Design review of the part shown in the three views and the two pictorial views. Dimensions are in mm from the part's minimum x, y and z. A direction names the side the tool comes from. Give positions to 0.01 mm unless a question says otherwise; leave off trailing zeros. Order: outer loops, then holes, each group sorted by start corner. A loop starts at its lowest first (then second) coordinate and runs counter-clockwise, first axis right, second up. Notation, with made-up numbers: (33.25, -9) - (72.25, -9) arc R11 ccw to (72.25, -2) - close; hole circle Ø3 at (85.25, 61). An arc over 180 degrees is marked (long way). Put each result on its own line as item: value.
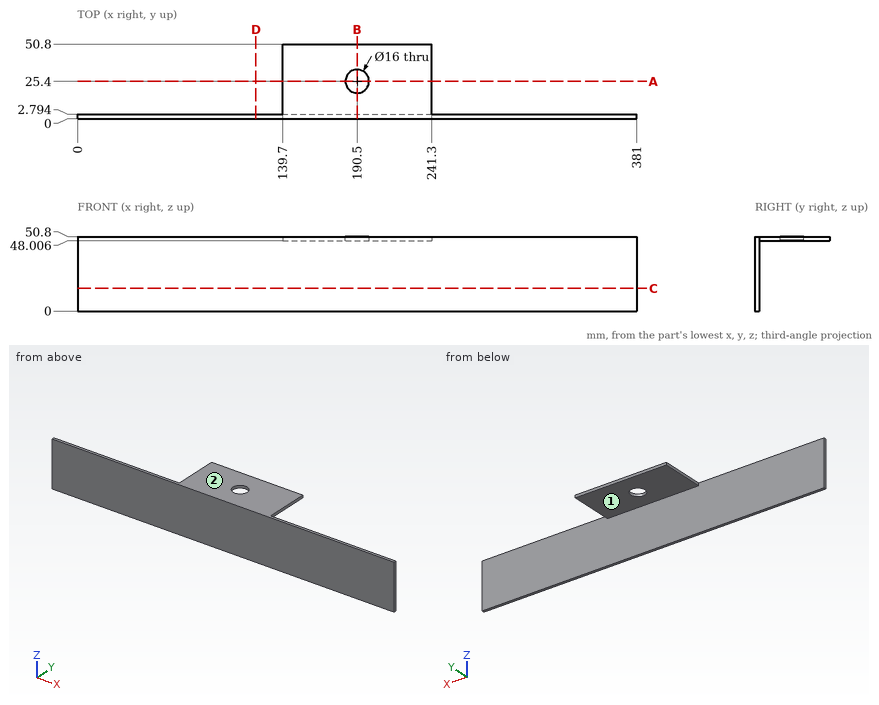
(1) Clearance check with flat-ended pins moving along their axes: pin 1 Ø14.5 at (x, y) = (190.5, 25.4) entering from -Z; pin 2 Ø4 at (x, z) = (326, 21.5) entering from +Y; pin 3 Ø0.8 at (y, z) = (36, 49) entering from +X; pin 4 Ø1.4 at (y, z) = (17.5, 49) entering from -X. State where each tip first meets the part, or that it passes through.
The answers:
pin 1: through
pin 2: y = 2.79
pin 3: x = 241.3
pin 4: x = 139.7
(2) For the marked faces 1 and 2, list the 3-axis set-ups (+Z, -Z, +X, -X, +Y, -Y) from which the entire face can be reached by the end or side of a thin tool; tool diameter is ignored.
The answers:
face 1: -Z, +X, -X, +Y
face 2: +Z, +X, -X, +Y, -Y
(3) Take a section at A-A, the plane y = 25.4. Write out the cut boundary in (x, z), then the cut area to 3 significant figures.
The answers:
outline: (139.7, 48.01) - (182.5, 48.01) - (182.5, 50.8) - (139.7, 50.8) - close; (198.5, 48.01) - (241.3, 48.01) - (241.3, 50.8) - (198.5, 50.8) - close
area: 239 mm^2
(4) Wall thickness on L1, parallel to Y at x = 190, z = 49; L2, parallel to Y at x = 314, z = 12; L3, parallel to Z at x = 219, y = 37: over which ranges is each line inside the solid? List them lowest first.
The answers:
L1: 0 to 17.42, 33.38 to 50.8
L2: 0 to 2.79
L3: 48.01 to 50.8
(5) Take a section at B-B, the plane x = 190.5. Write out the cut boundary in (y, z), then the cut area to 3 significant figures.
The answers:
outline: (0, 0) - (2.79, 0) - (2.79, 48.01) - (17.4, 48.01) - (17.4, 50.8) - (0, 50.8) - close; (33.4, 48.01) - (50.8, 48.01) - (50.8, 50.8) - (33.4, 50.8) - close
area: 231 mm^2
(6) Take a section at D-D, the plane x = 121.5. Write out the cut boundary in (y, z), then the cut area to 3 significant figures.
The answers:
outline: (0, 0) - (2.79, 0) - (2.79, 50.8) - (0, 50.8) - close
area: 142 mm^2
(7) Take a section at C-C, the plane z = 15.5. Write out the cut boundary in (x, y), then the cut area to 3 significant figures.
The answers:
outline: (0, 0) - (381, 0) - (381, 2.79) - (0, 2.79) - close
area: 1,060 mm^2
